Autodesk Inventor part; units mm, degrees
ref_plane "YZ Plane" through (0, 0, 0) normal (1, 0, 0) x (0, 1, 0)
ref_plane "XZ Plane" through (0, 0, 0) normal (0, 1, 0) x (-1, 0, 0)
ref_plane "XY Plane" through (0, 0, 0) normal (0, 0, 1) x (1, 0, 0)
sketch "Sketch1" plane through (0, 0, 0) normal (0, 1, 0) x (-1, 0, 0)
  circle A0 centre (0, 0) radius 1.5621
  dimension "d4" = 3.1242
extrude "Body" add sketch "Sketch1" along normal blind 31.75
sketch "Sketch2" plane through (0, 0, 0) normal (1, 0, 0) x (0, 1, 0)
  line L0 (31.75, -1.5621) -> (31.75, 1.5621)
  line L1 (31.75, 0) -> (31.75, -4.3688)
  line L2 (33.4772, 0) -> (31.75, 0)
  line L3 (33.4772, 0) -> (33.4772, -4.1656)
  arc A0 (33.4772, -4.1656) -> (34.4169, 0) centre (24.7141, 0) ccw
  line L4 (31.75, -4.3688) -> (33.4772, -4.1656)
  line L5 (33.4772, 0) -> (34.4169, 0)
  point P0 (0, 0)
  dimension "d5" = 4.3688
  dimension "d13" = 1.7272
  dimension "d57" = 4.1656
  dimension "d58" = 9.7028
  dimension "d59" = 0
revolve "Head" add sketch "Sketch2" angle 360 about axis through (0, 33.4772, 0) along (0, -1, 0)
sketch "Sketch6" plane through (0, 0, 0) normal (0, 0, 1) x (1, 0, 0)
  line L0 (0, 0) -> (-1.4859, 0)
  line L1 (1.5621, 0) -> (-1.5621, 0)
  line L2 (-1.4859, 0) -> (-2.4948, 1.0089)
  line L3 (-2.4948, 1.0089) -> (-2.9651, -1.2188)
  line L4 (-2.9651, -1.2188) -> (-1.4859, -1.2188)
  line L5 (-1.5621, 0) -> (-1.5621, 31.75)
  line L6 (-1.4859, -1.2188) -> (-1.4859, 0)
  line L7 (0, -3.9171) -> (0, 14.9707)
  point P0 (-1.5621, 0.0762)
  dimension "d49" = 1.4859
  dimension "d50" = 135
revolve "Tapered End" cut sketch "Sketch6" angle 360 about axis through (0, -10, 0) along (0, 1, 0)
sketch "Sketch7" plane through (0, 0, 0) normal (1, 0, 0) x (0, 1, 0)
  line L0 (31.75, 4.3688) -> (31.75, -4.3688)
  line L1 (33.0962, 0.6985) -> (33.0962, -0.6985)
  line L2 (33.0962, 0.6985) -> (35.1028, 0.6985)
  line L3 (35.1028, 0.6985) -> (35.1028, -0.6985)
  line L4 (35.1028, -0.6985) -> (33.0962, -0.6985)
  point P0 (0, 0)
  dimension "d61" = 1.397
  dimension "d62" = 0.6985
  dimension "d65" = 33.0962
  dimension "d66" = 2.0066
extrude "Flathead" cut sketch "Sketch7" against normal mid plane 12.7
properties part number "Screw 8-32 Nylon 1.250" material "VEX Nylon"
Model file for the job. Use its own axes, mm. A direction names the side the tool comes from. Round coordinates to 2 decimals unless told otherwise and drop trailing zeros. Write each loop counter-clockwise with the first axis right and the second up, starting at its lowest first coordinate (ties: lowest second). Pieces come first, ordered by that corner, then holes. Notation, with made-up numbers: M -3.5,28.25 L 35.5,28.25 A27 ccw 35.5,58.25 Z; hole C 2,14 d3. An arc over 180 degrees is marked long. Put each result on its own line as item: value.
Item 1: Cut at B-B (y = 8). List the corners of the cut face in (x, z).
Responses:
outline: C 0,0 d3.12
Item 2: Tool access for faces 1 (the flat face through (0, 33.096, 0)), 2 (the cylindrical face through (-1.49, 15.69, -0.47)): list every direction of +Z, -Z, +X, -X, +Y, -Y with a clear straight run to the whole face (end or side of a thin tool).
Responses:
face 1: +X, -X, +Y
face 2: -Y
Item 3: Flat gauge pins, fed straight in: P1, Ø1.4, axis at x = 1, y = 33.5, coming from the +Z side; P2, Ø4, axis at y = 5.5, z = 0.5, coming from the +X side; P3, Ø5, axis at x = 1.5, y = 6, coming from the +Z side. Where does each tip first touch, or does it go through?
Responses:
P1: z = 4.19
P2: x = 1.56
P3: z = 1.56
Item 4: Cut at A-A (z = 0). List the corners of the cut face in (x, y), and give its area (3 significant figures).
Responses:
outline: M -4.37,31.75 L -1.56,31.75 L -1.56,0.08 L -1.49,0 L 1.49,0 L 1.56,0.08 L 1.56,31.75 L 4.37,31.75 L 4.21,33.1 L -4.21,33.1 Z
area: 111 mm²
Item 5: Probe L1, parallel to Y at x = 3.75, z = -0.25; L2, parallel to X at y = 2, z = 0.5; L3, parallel to Y at x = 1.25, z = -0.25. List the from-to ranges inside material, lowest first. Write a range as from..to.
Responses:
L1: 31.75..33.1
L2: -1.48..1.48
L3: 0..33.1
Item 6: Mould opens along Z. For faces 3 (the conical face through (-4.12, 32.99, 0.92)), 4 (the flat face through (0, 0, 0)), 5 (the flat face through (0, 34, -0.698)) say: +Z half, -Z half, draft (parallel to the pull), parting line (faces both ways), or undercut.
Responses:
face 3: parting line
face 4: draft
face 5: undercut
